from build123d import *

# Parameters (mm, degrees)
BOSS_EXTRUDE1_DEPTH = 11
SKETCH2_R           = 4.75
CUT_EXTRUDE1_DEPTH  = 5
CUT_EXTRUDE2_START  = -5
SKETCH2_3_R         = 2.75
CUT_EXTRUDE2_DEPTH  = 87.961948653


with BuildPart() as part:
    # Profile → Boss-Extrude1 (new body)
    with BuildSketch(Plane.XY):
        with BuildLine():
            Line((0, 33), (9, 33))
            Line((9, 33), (9.5, 33.288675135))
            ThreePointArc((9.5, 33.288675135), (10.866025404, 32.922649731), (10.5, 31.556624327))
            Line((10.5, 31.556624327), (10, 31.267949192))
            Line((10, 31.267949192), (10, 23.732050808))
            Line((10, 23.732050808), (10.5, 23.443375673))
            ThreePointArc((10.5, 23.443375673), (10.866025404, 22.077350269), (9.5, 21.711324865))
            Line((9.5, 21.711324865), (9, 22))
            Line((9, 22), (0, 22))
            Line((0, 22), (0, 0))
            Line((0, 0), (80, 0))
            Line((80, 0), (80, 22))
            Line((80, 22), (71, 22))
            Line((71, 22), (70.5, 21.711324865))
            ThreePointArc((70.5, 21.711324865), (69.133974596, 22.077350269), (69.5, 23.443375673))
            Line((69.5, 23.443375673), (70, 23.732050808))
            Line((70, 23.732050808), (70, 31.267949192))
            Line((70, 31.267949192), (69.5, 31.556624327))
            ThreePointArc((69.5, 31.556624327), (69.133974596, 32.922649731), (70.5, 33.288675135))
            Line((70.5, 33.288675135), (71, 33))
            Line((71, 33), (80, 33))
            Line((80, 33), (80, 44))
            Line((80, 44), (0, 44))
            Line((0, 44), (0, 33))
        make_face()
    extrude(amount=BOSS_EXTRUDE1_DEPTH)

    # Sketch2 → Cut-Extrude1 (cut)
    with BuildSketch(Plane.XY.offset(11)):
        with Locations((40, 11)):
            Circle(SKETCH2_R)
    extrude(amount=-CUT_EXTRUDE1_DEPTH, mode=Mode.SUBTRACT)

    # Sketch2<3> → Cut-Extrude2 (cut, through all)
    with BuildSketch(Plane.XY.offset(11).offset(CUT_EXTRUDE2_START)):
        with Locations((40, 11)):
            Circle(SKETCH2_3_R)
    extrude(amount=-CUT_EXTRUDE2_DEPTH, mode=Mode.SUBTRACT)


solid = part.part
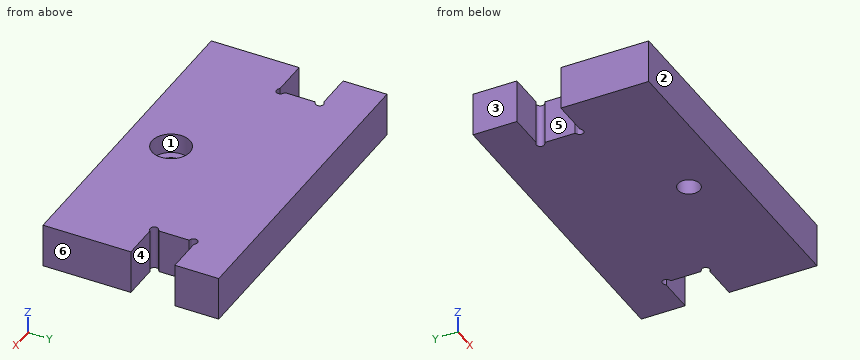
For this review, take the finished solid that the model builds, in its own axes (mm). Face numbers are marked on the shaded views. A direction names the side the tool comes from. Round coordinates to 2 decimals unless told otherwise and drop trailing zeros. Order: outer loops, then holes, each group sorted by start corner. A loop starts at its lowest first (then second) coordinate and runs counter-clockwise, first axis right, second up. Notation, with made-up numbers: (-33, 48.5) -> (-9, 48.5) arc R31 cw to (-9, 77.5) -> close; hole circle Ø4 at (27, 34). An arc over 180 degrees is marked (long way). Put each result on its own line as item: value.
Q1. Insertion check: pin 1 Ø6 at (x, y) = (70, 19.5) entering from -Z; pin 2 Ø7.5 at (x, y) = (39.5, 11) entering from +Z; pin 3 Ø2 at (y, z) = (29.5, 9.5) entering from -X. Each pin has a flat end and moves straight along its axis. Give the tip position at first contact, or say it passes through.
Check result:
pin 1: z = 0
pin 2: z = 6
pin 3: x = 10
Q2. Add section B-B on x = 40. Write out the cut boundary in (y, z), plus the area to 4 significant figures.
Check result:
outline: (0, 0) -> (8.25, 0) -> (8.25, 6) -> (6.25, 6) -> (6.25, 11) -> (0, 11) -> close; (13.75, 0) -> (44, 0) -> (44, 11) -> (15.75, 11) -> (15.75, 6) -> (13.75, 6) -> close
area: 403.5 mm2
Q3. Mouldability with a two-part tool opening along X and no side actions: class the marked faces 1, 2 and 3 as pulls with the +X half, pulls with the -X half, needs draft (parallel to the pull), parting line crosses it, or undercut.
Check result:
face 1: undercut
face 2: needs draft
face 3: pulls with the -X half
Q4. Machinability: for the marked faces 4, 5 and 6, which of the approach directions +Z, -Z, +X, -X, +Y, -Y give a long, thin tool a straight path to every point of the face, cutting with its end or side? Answer none if there is none.
Check result:
face 4: +Z, -Z, +X
face 5: +Z, -Z, -X
face 6: +Z, -Z, +X, +Y, -Y
Q5. For probe 1 along Y at (x, z) = (73.5, 2); probe 2 along Y at (x, z) = (40, 9.6); probe 3 along X at (y, z) = (26.5, 7.25), list the stretches that pass through material, from the lowest coordinate up. Write a range as [from, to].
Check result:
probe 1: [0, 22], [33, 44]
probe 2: [0, 6.25], [15.75, 44]
probe 3: [10, 70]
Q6. Add section D-D on y = 30. Write out the cut boundary in (x, z), plus the area to 3 significant figures.
Check result:
outline: (10, 0) -> (70, 0) -> (70, 11) -> (10, 11) -> close
area: 660 mm2
Q7. Add section A-A on y = 11. Write out the cut boundary in (x, z).
Check result:
outline: (0, 0) -> (37.25, 0) -> (37.25, 6) -> (35.25, 6) -> (35.25, 11) -> (0, 11) -> close; (42.75, 0) -> (80, 0) -> (80, 11) -> (44.75, 11) -> (44.75, 6) -> (42.75, 6) -> close
Q8. Add section C-C on z = 6.75. Write out the cut boundary in (x, y).
Check result:
outline: (0, 0) -> (80, 0) -> (80, 22) -> (71, 22) -> (70.5, 21.71) arc R1 cw to (69.5, 23.44) -> (70, 23.73) -> (70, 31.27) -> (69.5, 31.56) arc R1 cw to (70.5, 33.29) -> (71, 33) -> (80, 33) -> (80, 44) -> (0, 44) -> (0, 33) -> (9, 33) -> (9.5, 33.29) arc R1 cw to (10.5, 31.56) -> (10, 31.27) -> (10, 23.73) -> (10.5, 23.44) arc R1 cw to (9.5, 21.71) -> (9, 22) -> (0, 22) -> close; hole circle Ø9.5 at (40, 11)
